from build123d import *

# Parameters (mm, degrees)
BOSS_EXTRUDE1_DEPTH  = 3.175
M4_CLEARANCE_HOLE1_D = 4.5


with BuildPart() as part:
    # Sketch1 → Boss-Extrude1 (new body)
    with BuildSketch(Plane(origin=(0, 0, 0), x_dir=(1, 0, 0), z_dir=(0, 1, 0))):
        Polygon((-98.425, 50.8), (-50.8, 98.425), (50.8, 98.425), (98.425, 50.8), (98.425, -50.8), (50.8, -98.425), (-50.8, -98.425), (-98.425, -50.8), align=None)
    extrude(amount=BOSS_EXTRUDE1_DEPTH)

    # M4 Clearance Hole1 (through all)
    with Locations(Plane(origin=(-15, 3.175, -87.425), x_dir=(0, 0, 1), z_dir=(0, 1, 0))):
        with Locations((0, 0), (28, 0), (28, 30), (0, 30)):
            m4_clearance_hole1 = Hole(M4_CLEARANCE_HOLE1_D / 2)

    # Mirror1: M4 Clearance Hole1 across plane
    add(m4_clearance_hole1.mirror(Plane.XY), mode=Mode.SUBTRACT)


solid = part.part
Can you work these out from the model? Positions are in its coordinate system, mm. Give positions to 0.01 mm unless a question says otherwise; leave off trailing zeros. Loops run counter-clockwise (first coordinate to the right, second up) from the corner with the lowest first, then second, coordinate; pieces in that order, holes last. Notation, with made-up numbers: (-18, -10.5) - (5, -10.5) arc R16 cw to (5, 1.5) - close; hole circle Ø8 at (72, -0.5). An arc over 180 degrees is marked (long way). One line per item, written item: value.
(1) I need wall thicknesses on line 1 along X through (y, z) = (2.35, 59) (1 decimal); line 2 along Z through (x, y) = (-70, 2.7) (3 decimals); line 3 along Z through (x, y) = (56.5, 2.45) (3 decimals). Which ranges of each line are inside material? Lowest first, please.
Verdict:
line 1: -90.2 to -17.2, -12.8 to 12.8, 17.2 to 90.2
line 2: -79.225 to 79.225
line 3: -92.725 to 92.725
(2) If we mould it in two halves opening along Z, with no side actions, what happens to faces 1 (the face through (1, 0, -1)), 2 (the face through (74.279, 1.565, -74.946)), 3 (the face through (14.138, 1.565, -61.503))? For each: released by +Z, released by -Z, zero draft, split by the parting line, or undercut.
Verdict:
face 1: zero draft
face 2: released by -Z
face 3: undercut
(3) I'm going to push flat-ended pins straight in: pin 1 (7 mm diameter, centred on x = -15, z = -87.425, fed in from -Y); pin 2 (4 mm diameter, centred on x = 15, z = -87.425, fed in from -Y). Where does each tip first touch, or does it pass through?
Verdict:
pin 1: y = 0
pin 2: through
(4) If we section it at A-A, the plane x = 15: List the corners of the cut face in (y, z) for me (3 decimals), plus the area to 3 significant figures.
Verdict:
outline: (0, -98.425) - (3.175, -98.425) - (3.175, -89.675) - (0, -89.675) - close; (0, -85.175) - (3.175, -85.175) - (3.175, -61.675) - (0, -61.675) - close; (0, -57.175) - (3.175, -57.175) - (3.175, 57.175) - (0, 57.175) - close; (0, 61.675) - (3.175, 61.675) - (3.175, 85.175) - (0, 85.175) - close; (0, 89.675) - (3.175, 89.675) - (3.175, 98.425) - (0, 98.425) - close
area: 568 mm^2
(5) If we section it at C-C, the plane x = -64: List the corners of the cut face in (y, z) for me (3 decimals), plus the area to 3 significant figures.
Verdict:
outline: (0, -85.225) - (3.175, -85.225) - (3.175, 85.225) - (0, 85.225) - close
area: 541 mm^2
(6) If we section it at B-B, the plane y = 1.4: State how many separate pieces and enclosed holes the cut face has, plus the area to 3 significant figures.
Verdict:
separate pieces: 1
enclosed holes: 8
area: 34,100 mm^2
